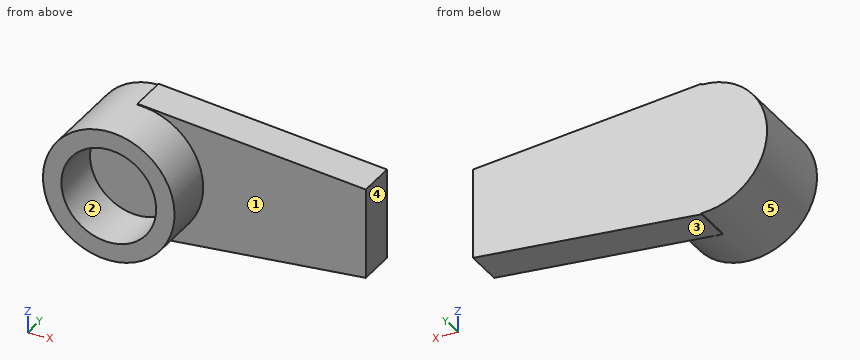
```python
from build123d import *

# Parameters (mm, degrees)
BOSS_EXTRUDE1_START = 19.3
SKETCH1_R           = 3.4
BOSS_EXTRUDE1_DEPTH = 2.35
BOSS_EXTRUDE2_START = 20.65
BOSS_EXTRUDE2_DEPTH = 1
CUT_EXTRUDE1_START  = 18.3
SKETCH3_R           = 2.45
CUT_EXTRUDE1_DEPTH  = 1.35


with BuildPart() as part:
    # Sketch1 → Boss-Extrude1 (new, symmetric)
    with BuildSketch(Plane(origin=(0, 0, 0), x_dir=(1, 0, 0), z_dir=(0, 1, 0)).offset(BOSS_EXTRUDE1_START)):
        with Locations(Location((0, 0, 0), (0, 0, 90))):
            Circle(SKETCH1_R)
    extrude(amount=BOSS_EXTRUDE1_DEPTH, both=True)

    # Sketch2 → Boss-Extrude2 (add, symmetric)
    with BuildSketch(Plane(origin=(0, 0, 0), x_dir=(1, 0, 0), z_dir=(0, 1, 0)).offset(BOSS_EXTRUDE2_START)):
        Polygon((0, 3.453116188), (11.8, 2.337687781), (11.8, -2.337687781), (0, -3.453116188), align=None)
    extrude(amount=BOSS_EXTRUDE2_DEPTH, both=True)

    # Sketch3 → Cut-Extrude1 (cut, symmetric)
    with BuildSketch(Plane(origin=(0, 0, 0), x_dir=(1, 0, 0), z_dir=(0, 1, 0)).offset(CUT_EXTRUDE1_START)):
        with Locations(Location((0, 0, 0), (0, 0, 270))):
            Circle(SKETCH3_R)
    extrude(amount=CUT_EXTRUDE1_DEPTH, both=True, mode=Mode.SUBTRACT)


solid = part.part
```
The listing builds one solid part. Answer for the finished solid, in the listing's coordinates (mm). Face numbers are marked on the shaded views. A direction names the side the tool comes from. Round coordinates to 2 decimals unless told otherwise and drop trailing zeros. Loops run counter-clockwise (first coordinate to the right, second up) from the corner with the lowest first, then second, coordinate; pieces in that order, holes last. Notation, with made-up numbers: (63, 36) - (116, 36) arc R16 ccw to (116, 54) - close; hole circle Ø7 at (64.25, 82). An arc over 180 degrees is marked (long way). Return JSON: item names as keys, results as strings. Group by question number.
1. The part is cut by section C-C on x = 1.25. Determine the outline of the cut face in (y, z).
2. Consider probe 1 along X at (y, z) = (17.95, 0); probe 2 along Y at (x, z) = (1.5, -0.5); probe 3 along X at (y, z) = (18.35, -1). Determine where each line is inside the solid, lowest interval first.
3. Which of the six approach directions +Z, -Z, +X, -X, +Y, -Y give full straight-line access (tool end or side, diameter ignored) to the marked faces 4 and 5?
4. The mould has two halves that part along X. Classify the marked faces 1, 2 and 3: pulls with the +X half, pulls with the -X half, needs draft (parallel to the pull), parting line crosses it, or undercut.
5. The part is cut by section D-D on y = 21.35. Determine the outline of the cut face in (x, z), then the cut area to 3 significant figures.
6. The part is cut by section A-A on y = 17.2. Determine the outline of the cut face in (x, z), then the cut area to 3 significant figures.
7. Each of these flat-tipped pins is pushed along its axis until it touches: P1, Ø1, axis at x = 3, y = 18.5, coming from the -Z side; P2, Ø2, axis at x = 6.5, z = 1, coming from the -Y side; P3, Ø2, axis at y = 20.5, z = 2.5, coming from the -X side. Where does it stop, or does it pass through?
8. The part is cut by section B-B on z = 0. Determine the outline of the cut face in (x, y), then the cut area to 3 significant figures.
Resolved:
{
 "1": {"outline": "(16.95, -3.16) - (19.65, -3.16) - (19.65, -3.33) - (21.65, -3.33) - (21.65, 3.33) - (19.65, 3.33) - (19.65, 3.16) - (16.95, 3.16) - (16.95, 2.11) - (19.65, 2.11) - (19.65, -2.11) - (16.95, -2.11) - close"},
 "2": {"probe 1": "x = -3.4 to -2.45, 2.45 to 3.4", "probe 2": "y = 19.65 to 21.65", "probe 3": "x = -3.25 to -2.24, 2.24 to 3.25"},
 "3": {"face 4": "+Z, -Z, +X, +Y, -Y", "face 5": "-Y"},
 "4": {"face 1": "needs draft", "face 2": "undercut", "face 3": "pulls with the +X half"},
 "5": {"outline": "(0, -3.45) - (11.8, -2.34) - (11.8, 2.34) - (0, 3.45) - (0, 3.4) arc R3.4 ccw to (0, -3.4) - close", "area": "86.5 mm²"},
 "6": {"outline": "circle Ø6.8 at (0, 0); hole circle Ø4.9 at (0, 0)", "area": "17.5 mm²"},
 "7": {"P1": "stops at z = -2.3", "P2": "stops at y = 19.65", "P3": "stops at x = -3.05"},
 "8": {"outline": "(-3.4, 16.95) - (-2.45, 16.95) - (-2.45, 19.65) - (2.45, 19.65) - (2.45, 16.95) - (3.4, 16.95) - (3.4, 19.65) - (11.8, 19.65) - (11.8, 21.65) - (-3.4, 21.65) - close", "area": "35.5 mm²"}
}
